Verification items for the finished model (mm, model axes). A direction names the side the tool comes from. Round coordinates to 2 decimals unless told otherwise and drop trailing zeros. Order: outer loops, then holes, each group sorted by start corner. A loop starts at its lowest first (then second) coordinate and runs counter-clockwise, first axis right, second up. Notation, with made-up numbers: M 18,54.5 L 42,54.5 A11 cw 42,60.5 Z; hole C 21.5,28.25 d6. An arc over 180 degrees is marked long. Use CSV: the item, a comma, the result in double quotes. Start each with the question number.
Q1. Scan lines: line 1 (X direction, y = -0.1, z = 0); line 2 (X direction, y = -1.5, z = -1.75); line 3 (Z direction, x = 2, y = -0.85). Record each from-to range of solid material in increasing order.
Q2. Sectioned sample at B-B (y = 0). Enter the section's corners in (x, z), and give its area (3 significant figures).
Q3. Sectioned sample at C-C (x = 19.5). Enter the section's corners in (y, z).
Q4. Mould release check, pull along Z, two halves, no side actions. Record for faces 3 (the face through (20, 1.2, 1.2)), 4 (the face through (2, 0, 1)), 5 (the face through (20.99, -4.88, 1.08)): +Z half, -Z half, draft (parallel to the pull), parting line (faces both ways), or undercut.
Q5. Set-up check for faces 1 (the face through (0, 0, 0)), 2 (the face through (9.86, 0.07, 1.5)): record each of +Z, -Z, +X, -X, +Y, -Y from which the full face is reachable in a straight line by a thin tool's end or side.
Q6. Sectioned sample at A-A (z = 0). Enter the section's corners in (x, y).
Q7. Sectioned sample at D-D (y = 4). Enter the section's corners in (x, z), and give its area (3 significant figures).
Q8. Gauge pin test, flat ends, axial feed: pin 1 Ø1 at (y, z) = (2.5, 2) entering from -X; pin 2 Ø2.5 at (x, z) = (2, 0) entering from +Y; pin 3 Ø2.5 at (x, z) = (7.5, 0) entering from -Y. Record the tip position at first contact, or that the pin passes through.
```python
from build123d import *

# Parameters (mm, degrees)
SKETCH1_R               = 1.5
BOSS_EXTRUDE4_DEPTH     = 20
SKETCH5_R               = 5
BOSS_EXTRUDE5_DEPTH     = 2
CUT_EXTRUDE1_DEPTH      = 24.108440017
CUT_EXTRUDE1_DEPTH_BACK = 24.108440017
SKETCH6_R               = 1


with BuildPart() as part:
    # Sketch1 → Boss-Extrude4 (new body)
    with BuildSketch(Plane(origin=(0, 0, 0), x_dir=(0, 0, -1), z_dir=(1, 0, 0))):
        Circle(SKETCH1_R)
    extrude(amount=BOSS_EXTRUDE4_DEPTH)

    # Sketch5 → Boss-Extrude5 (add)
    with BuildSketch(Plane(origin=(20, 0, 0), x_dir=(0, 0, -1), z_dir=(1, 0, 0))):
        Circle(SKETCH5_R)
    extrude(amount=BOSS_EXTRUDE5_DEPTH)

    # Sketch6 → Cut-Extrude1 (cut, two sides: drawn at the far end of the back side and taken through both)
    with BuildSketch(Plane(origin=(0, 0, 0), x_dir=(1, 0, 0), z_dir=(0, 1, 0)).offset(-CUT_EXTRUDE1_DEPTH_BACK)):
        with Locations(Location((2, 0, 0), (0, 0, 270))):
            Circle(SKETCH6_R)
        with Locations(Location((7.5, 0, 0), (0, 0, 270))):
            Circle(SKETCH6_R)
    extrude(amount=CUT_EXTRUDE1_DEPTH + CUT_EXTRUDE1_DEPTH_BACK, mode=Mode.SUBTRACT)


solid = part.part
```
Verdict:
1,line 1,"x = 0 to 1, 3 to 6.5, 8.5 to 22"
1,line 2,"x = 20 to 22"
1,line 3,"z = -1.24 to -1, 1 to 1.24"
2,outline,"M 0,-1.5 L 20,-1.5 L 20,-5 L 22,-5 L 22,5 L 20,5 L 20,1.5 L 0,1.5 Z; hole C 2,0 d2; hole C 7.5,0 d2"
2,area,"73.7 mm²"
3,outline,"C 0,0 d3"
4,face 3,"draft"
4,face 4,"undercut"
4,face 5,"parting line"
5,face 1,"+Z, -Z, -X, +Y, -Y"
5,face 2,"-X"
6,outline,"M 0,-1.5 L 1,-1.5 L 1,1.5 L 0,1.5 Z; M 3,-1.5 L 6.5,-1.5 L 6.5,1.5 L 3,1.5 Z; M 8.5,-1.5 L 20,-1.5 L 20,-5 L 22,-5 L 22,5 L 20,5 L 20,1.5 L 8.5,1.5 Z"
7,outline,"M 20,-3 L 22,-3 L 22,3 L 20,3 Z"
7,area,"12.0 mm²"
8,pin 1,"stops at x = 20"
8,pin 2,"stops at y = 1.5"
8,pin 3,"stops at y = -1.5"
